Geometry: final body of the model. Coordinates: model frame, mm. Face numbers are marked on the shaded views. A direction names the side the tool comes from. Coordinates: 2 decimals unless noted, no trailing zeros. Loops run counter-clockwise (first coordinate to the right, second up) from the corner with the lowest first, then second, coordinate; pieces in that order, holes last. Notation, with made-up numbers: (-16.75, -4.5) - (6.25, -4.5) arc R19 cw to (6.25, 0.5) - close; hole circle Ø7 at (27.5, -28.75). An arc over 180 degrees is marked (long way). Return JSON: item names as keys, results as strings.
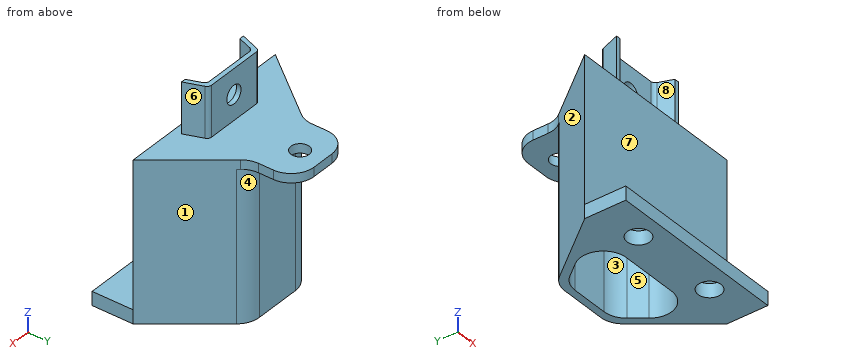
from build123d import *

# Parameters (mm, degrees)
SKETCH1_W               = 40
SKETCH1_H               = 25
SKETCH1_R               = 2.5
BOSS_EXTRUDE1_DEPTH     = 34.73
BOSS_EXTRUDE2_DEPTH     = 11
FILLET3_R               = 1
SKETCH5_W               = 15
SKETCH5_H               = 2
BOSS_EXTRUDE3_DEPTH     = 10
SKETCH8_R               = 2
CUT_EXTRUDE4_DEPTH      = 12
CUT_EXTRUDE4_DEPTH_BACK = 35.73
SKETCH10_W              = 40
SKETCH10_H              = 9
CUT_EXTRUDE5_DEPTH      = 22
CUT_EXTRUDE7_DEPTH      = 35.73
SKETCH7_R               = 2
CUT_EXTRUDE9_DEPTH      = 22
CUT_EXTRUDE8_DEPTH      = 22
FILLET7_R               = 5
FILLET8_R               = 5
FILLET9_R               = 5
FILLET10_R              = 5
FILLET11_R              = 5
FILLET12_R              = 5
FILLET13_R              = 5
FILLET14_R              = 5
FILLET15_R              = 5
FILLET16_R              = 5
SKETCH15_W              = 40
SKETCH15_H              = 9
CUT_EXTRUDE10_DEPTH     = 9.73


with BuildPart() as part:
    # Sketch1 → Boss-Extrude1 (new body)
    with BuildSketch(Plane.XY):
        with Locations((20, 12.5)):
            Rectangle(SKETCH1_W, SKETCH1_H)
        with Locations((10, 5)):
            Circle(SKETCH1_R, mode=Mode.SUBTRACT)
        with Locations((30, 5)):
            Circle(SKETCH1_R, mode=Mode.SUBTRACT)
    extrude(amount=BOSS_EXTRUDE1_DEPTH)

    # Sketch2 → Boss-Extrude2 (add)
    with BuildSketch(Plane.XY.offset(34.73)):
        Polygon((27, 15.5), (13, 15.5), (11.289899283, 10.801536896), (12.289899283, 10.801536896), (13.636029766, 14.5), (26.363970234, 14.5), (27.710100717, 10.801536896), (28.710100717, 10.801536896), align=None)
    extrude(amount=BOSS_EXTRUDE2_DEPTH)

    # Fillet3
    fillet3_edges = [part.edges().sort_by_distance(p)[0] for p in [
        (13, 15.5, 40.23),
        (13.636029766, 14.5, 40.23),
        (26.363970234, 14.5, 40.23),
        (27, 15.5, 40.23),
    ]]
    fillet(fillet3_edges, radius=FILLET3_R)

    # Sketch5 → Boss-Extrude3 (add)
    with BuildSketch(Plane(origin=(0, 25, 0), x_dir=(1, 0, 0), z_dir=(0, 1, 0))):
        with Locations((20, -33.73)):
            Rectangle(SKETCH5_W, SKETCH5_H)
    extrude(amount=BOSS_EXTRUDE3_DEPTH)

    # Sketch8 → Cut-Extrude4 (cut, two sides)
    with BuildSketch(Plane.XY.offset(34.73)) as cut_extrude4_sk:
        with Locations((20, 30)):
            Circle(SKETCH8_R)
    extrude(amount=CUT_EXTRUDE4_DEPTH, mode=Mode.SUBTRACT)
    extrude(cut_extrude4_sk.sketch, amount=-CUT_EXTRUDE4_DEPTH_BACK, mode=Mode.SUBTRACT)

    # Sketch10 → Cut-Extrude5 (cut)
    with BuildSketch(Plane.XY.offset(34.73)):
        with Locations((20, 4.5)):
            Rectangle(SKETCH10_W, SKETCH10_H)
    extrude(amount=-CUT_EXTRUDE5_DEPTH, mode=Mode.SUBTRACT)

    # Sketch12 → Cut-Extrude7 (cut, through all)
    with BuildSketch(Plane.XY.offset(34.73)):
        Polygon((12.5, 25), (0, 9), (0, 25), align=None)
        Polygon((27.5, 25), (40, 9), (40, 25), align=None)
    extrude(amount=-CUT_EXTRUDE7_DEPTH, mode=Mode.SUBTRACT)

    # Sketch7 → Cut-Extrude9 (cut)
    with BuildSketch(Plane.XZ.offset(-14.5)):
        with Locations((20, 40.23)):
            Circle(SKETCH7_R)
    extrude(amount=-CUT_EXTRUDE9_DEPTH, mode=Mode.SUBTRACT)

    # Sketch14 → Cut-Extrude8 (cut)
    with BuildSketch(Plane(origin=(0, 0, 0), x_dir=(-1, 0, 0), z_dir=(0, 0, -1))):
        Polygon((-36.656713145, 10.5), (-26.5, 23.5), (-13.5, 23.5), (-3.343286855, 10.5), align=None)
    extrude(amount=-CUT_EXTRUDE8_DEPTH, mode=Mode.SUBTRACT)

    # Fillet7
    fillet7_edges = [part.edges().sort_by_distance(p)[0] for p in [
        (27.5, 25, 16.365),
    ]]
    fillet(fillet7_edges, radius=FILLET7_R)

    # Fillet8
    fillet8_edges = [part.edges().sort_by_distance(p)[0] for p in [
        (27.5, 25, 33.73),
    ]]
    fillet(fillet8_edges, radius=FILLET8_R)

    # Fillet9
    fillet9_edges = [part.edges().sort_by_distance(p)[0] for p in [
        (12.5, 25, 16.365),
    ]]
    fillet(fillet9_edges, radius=FILLET9_R)

    # Fillet10
    fillet10_edges = [part.edges().sort_by_distance(p)[0] for p in [
        (12.5, 25, 33.73),
    ]]
    fillet(fillet10_edges, radius=FILLET10_R)

    # Fillet11
    fillet11_edges = [part.edges().sort_by_distance(p)[0] for p in [
        (3.343286855, 10.5, 11),
    ]]
    fillet(fillet11_edges, radius=FILLET11_R)

    # Fillet12
    fillet12_edges = [part.edges().sort_by_distance(p)[0] for p in [
        (36.656713145, 10.5, 11),
    ]]
    fillet(fillet12_edges, radius=FILLET12_R)

    # Fillet13
    fillet13_edges = [part.edges().sort_by_distance(p)[0] for p in [
        (26.5, 23.5, 11),
    ]]
    fillet(fillet13_edges, radius=FILLET13_R)

    # Fillet14
    fillet14_edges = [part.edges().sort_by_distance(p)[0] for p in [
        (13.5, 23.5, 11),
    ]]
    fillet(fillet14_edges, radius=FILLET14_R)

    # Fillet15
    fillet15_edges = [part.edges().sort_by_distance(p)[0] for p in [
        (27.5, 35, 33.73),
    ]]
    fillet(fillet15_edges, radius=FILLET15_R)

    # Fillet16
    fillet16_edges = [part.edges().sort_by_distance(p)[0] for p in [
        (12.5, 35, 33.73),
    ]]
    fillet(fillet16_edges, radius=FILLET16_R)

    # Sketch15 → Cut-Extrude10 (cut)
    with BuildSketch(Plane.XY.offset(12.73)):
        with Locations((20, 4.5)):
            Rectangle(SKETCH15_W, SKETCH15_H)
    extrude(amount=-CUT_EXTRUDE10_DEPTH, mode=Mode.SUBTRACT)


solid = part.part
Item 1: Reachability of the marked faces 4, 5, 6, 7 and 8 from +Z, -Z, +X, -X, +Y, -Y: full face, straight path, thin tool, end or side. Return the list, or none.
Worked out:
{"face 4": "-Z, +X, +Y", "face 5": "-Z", "face 6": "+Z, +X, +Y", "face 7": "+Z, +X, -X, -Y", "face 8": "+Z, -Y"}
Item 2: Section query D-D, the plane y = 31. Return loops of the section in (x, z).
Worked out:
{"outline": "(12.6, 32.73) - (18.27, 32.73) - (18.27, 34.73) - (12.6, 34.73) - close; (21.73, 32.73) - (27.4, 32.73) - (27.4, 34.73) - (21.73, 34.73) - close"}
Item 3: Section query C-C, the plane x = 37. Return loops of the section in (y, z), and give its area (3 significant figures).
Worked out:
{"outline": "(0, 0) - (12.84, 0) - (12.84, 34.73) - (9, 34.73) - (9, 3) - (0, 3) - close", "area": "160 mm^2"}
Item 4: First-contact query: pin 1 Ø2 at (x, z) = (19, 29) entering from +Y; pin 2 Ø16 at (x, z) = (29.5, 11.5) entering from -Y; pin 3 Ø6.5 at (x, y) = (20, 30) entering from +Z; pin 4 Ø3 at (y, z) = (6, 10.5) entering from -X. Flat tips, straight axial feed; report the tip coordinate or a pass-through.
Worked out:
{"pin 1": "y = 25", "pin 2": "y = 9", "pin 3": "z = 34.73", "pin 4": "through"}
Item 5: Section query B-B, the plane z = 12.5. Return loops of the section in (x, y).
Worked out:
{"outline": "(0, 9) - (40, 9) - (29, 23.08) arc R5 ccw to (25.06, 25) - (14.94, 25) arc R5 ccw to (11, 23.08) - close; hole (9.65, 18.58) arc R5 ccw to (13.59, 10.5) - (26.41, 10.5) arc R5 ccw to (30.35, 18.58) - (28, 21.58) arc R5 ccw to (24.06, 23.5) - (15.94, 23.5) arc R5 ccw to (12, 21.58) - close"}
Item 6: Mould query, pull axis X, two halves, no side actions, for the marked faces 1, 2 and 3. Classes: +X half, -X half, draft (parallel to the pull), parting line (faces both ways), or undercut.
Worked out:
{"face 1": "+X half", "face 2": "-X half", "face 3": "undercut"}
Item 7: Section query A-A, the plane x = 20. Return loops of the section in (y, z).
Worked out:
{"outline": "(0, 0) - (10.5, 0) - (10.5, 22) - (23.5, 22) - (23.5, 0) - (25, 0) - (25, 32.73) - (28, 32.73) - (28, 34.73) - (15.5, 34.73) - (15.5, 38.23) - (14.5, 38.23) - (14.5, 34.73) - (9, 34.73) - (9, 3) - (0, 3) - close; (14.5, 42.23) - (15.5, 42.23) - (15.5, 45.73) - (14.5, 45.73) - close; (32, 32.73) - (35, 32.73) - (35, 34.73) - (32, 34.73) - close"}
Item 8: Ray query, probe 1 along X at (y, z) = (5, 1.6); probe 2 along Z at (x, y) = (20, 15.05); probe 3 along Y at (x, z) = (10, 1.85). Return the intervals inside material, ascending. Write a range as from..to.
Worked out:
{"probe 1": "0..7.5, 12.5..27.5, 32.5..40", "probe 2": "22..38.23, 42.23..45.73", "probe 3": "0..2.5, 7.5..12.02, 19.02..21.8"}
